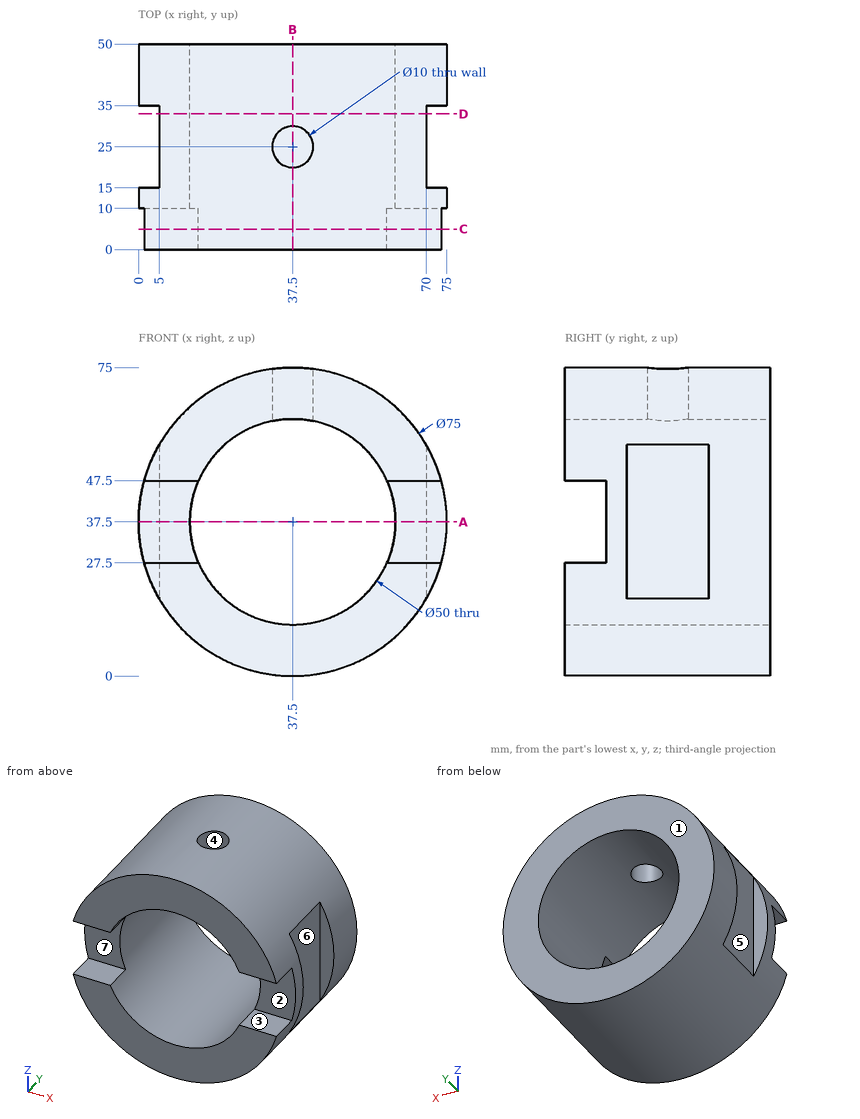
Here's the drawing with two shaded views (mm, measured from the low corner). I have some questions. A direction names the side the tool comes from. Give positions to 0.01 mm unless a question says otherwise; leave off trailing zeros. Order: outer loops, then holes, each group sorted by start corner. A loop starts at its lowest first (then second) coordinate and runs counter-clockwise, first axis right, second up.
Q1. Suppose I cut it at D-D, the plane y = 33. Write out the boundary of the cut face in (x, z).
Q2. I'm going to push flat-ended pins straight in: P1, Ø6, axis at y = 13.5, z = 20, coming from the -X side; P2, Ø1.5, axis at y = 7, z = 26, coming from the -X side; P3, Ø4, axis at y = 11, z = 52, coming from the -X side; P4, Ø10, axis at x = 33, z = 53.5, coming from the -Y side. Where does each tip first touch, or does it pass through?
Q3. Suppose I cut it at C-C, the plane y = 5. Write out the boundary of the cut face in (x, z).
Q4. If I drill on line 1 along Y through (x, z) = (3, 48); line 2 along Y through (x, z) = (37.5, 66.75); line 3 along Y through (x, z) = (62, 43), over which ranges is the centre line in solid material (lowest first)?
Q5. For the marked faces 5, 6 and 7, which set-ups out of +Z, -Z, +X, -X, +Y, -Y let a thin tool reach every point of the face, with its end or its side?
Q6. We'd pull the mould along Y, two halves only. Please class the marked faces 1, 2, 3 and 4: +Y half, -Y half, draft (parallel to the pull), parting line (faces both ways), or undercut.
Q7. Suppose I cut it at B-B, the plane x = 37.5. Write out the boundary of the cut face in (y, z), and give its area (4 significant figures).
Q8. Suppose I cut it at A-A, the plane z = 37.5. Write out the boundary of the cut face in (x, y).
Solution:
1. outline: (5, 18.79) arc R37.5 ccw to (70, 18.79) - (70, 56.21) arc R37.5 ccw to (5, 56.21) - close; hole circle Ø50 at (37.5, 37.5)
2. P1: stops at x = 2.92
2. P2: stops at x = 1.57
2. P3: stops at x = 2.14
2. P4: passes through
3. outline: (1.36, 27.5) arc R37.5 ccw to (73.64, 27.5) - (60.41, 27.5) arc R25 cw to (14.59, 27.5) - close; (1.36, 47.5) - (14.59, 47.5) arc R25 cw to (60.41, 47.5) - (73.64, 47.5) arc R37.5 ccw to start
4. line 1: y = 0 to 15, 35 to 50
4. line 2: y = 0 to 20, 30 to 50
4. line 3: y = 10 to 50
5. face 5: +Z, -Z, -X
5. face 6: +Z, -Z, +X
5. face 7: +X, -X, -Y
6. face 1: +Y half
6. face 2: -Y half
6. face 3: draft
6. face 4: undercut
7. outline: (0, 0) - (50, 0) - (50, 12.5) - (0, 12.5) - close; (0, 62.5) - (20, 62.5) - (20, 75) - (0, 75) - close; (30, 62.5) - (50, 62.5) - (50, 75) - (30, 75) - close
7. area: 1,125 mm2
8. outline: (0, 10) - (12.5, 10) - (12.5, 50) - (0, 50) - (0, 35) - (5, 35) - (5, 15) - (0, 15) - close; (62.5, 10) - (75, 10) - (75, 15) - (70, 15) - (70, 35) - (75, 35) - (75, 50) - (62.5, 50) - close
